Verification items for the finished model (mm, model axes). Face numbers are marked on the shaded views. A direction names the side the tool comes from. Coordinates: 2 decimals unless noted, no trailing zeros. Write each loop counter-clockwise with the first axis right and the second up, starting at its lowest first coordinate (ties: lowest second). Pieces come first, ordered by that corner, then holes. Notation, with made-up numbers: (-0.75, -10) -> (29.25, -10) arc R24 cw to (29.25, 8) -> close; hole circle Ø7 at (-0.5, -27.5). An arc over 180 degrees is marked (long way). Answer in a Markdown table with one row per item.
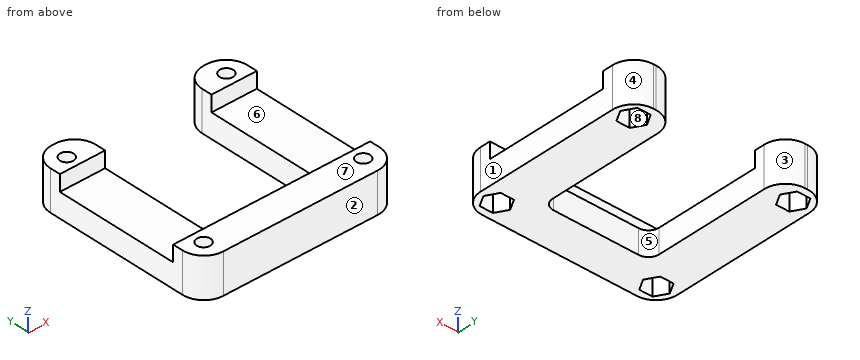
```python
from build123d import *

# Parameters (mm, degrees)
F0_R     = 1.6256
F1_DEPTH = 9.525
F2_W     = 46.99
F2_H     = 29.464
F3_DEPTH = 3.81
F5_DEPTH = 4.064


with BuildPart() as f1:
    # F0 (on Top) → F1 (new body)
    with BuildSketch(Plane.XY):
        with BuildLine():
            ThreePointArc((23.495, 17.145), (22.007102, 20.737102), (18.415, 22.225))
            Line((18.415, 22.225), (17.78, 22.225))
            ThreePointArc((17.78, 22.225), (14.187898, 20.737102), (12.7, 17.145))
            Line((12.7, 17.145), (12.7, -10.16))
            ThreePointArc((12.7, -10.16), (11.956051, -11.956051), (10.16, -12.7))
            Line((10.16, -12.7), (-10.16, -12.7))
            ThreePointArc((-10.16, -12.7), (-11.956051, -11.956051), (-12.7, -10.16))
            Line((-12.7, -10.16), (-12.7, 17.145))
            ThreePointArc((-12.7, 17.145), (-14.187898, 20.737102), (-17.78, 22.225))
            Line((-17.78, 22.225), (-18.415, 22.225))
            ThreePointArc((-18.415, 22.225), (-22.007102, 20.737102), (-23.495, 17.145))
            Line((-23.495, 17.145), (-23.495, -17.145))
            ThreePointArc((-23.495, -17.145), (-22.007102, -20.737102), (-18.415, -22.225))
            Line((-18.415, -22.225), (18.415, -22.225))
            ThreePointArc((18.415, -22.225), (22.007102, -20.737102), (23.495, -17.145))
            Line((23.495, -17.145), (23.495, 17.145))
        make_face()
        with Locations((-19.05, -17.78)):
            Circle(F0_R, mode=Mode.SUBTRACT)
        with Locations((19.05, -17.78)):
            Circle(F0_R, mode=Mode.SUBTRACT)
        with Locations((-19.05, 17.78)):
            Circle(F0_R, mode=Mode.SUBTRACT)
        with Locations((19.05, 17.78)):
            Circle(F0_R, mode=Mode.SUBTRACT)
    extrude(amount=F1_DEPTH)

    # F2 (on face) → F3 (cut)
    with BuildSketch(Plane.XY.offset(9.525)):
        Rectangle(F2_W, F2_H)
    extrude(amount=-F3_DEPTH, mode=Mode.SUBTRACT)

    # F4 (on face) → F5 (cut)
    with BuildSketch(Plane(origin=(0, 0, 0), x_dir=(1, 0, 0), z_dir=(0, 0, -1))):
        Polygon((17.466213, -15.0368), (15.882425, -17.78), (17.466213, -20.5232), (20.633787, -20.5232), (22.217575, -17.78), (20.633787, -15.0368), align=None)
        Polygon((-17.466213, -15.0368), (-20.633787, -15.0368), (-22.217575, -17.78), (-20.633787, -20.5232), (-17.466213, -20.5232), (-15.882425, -17.78), align=None)
        Polygon((15.882425, 17.78), (17.466213, 15.0368), (20.633787, 15.0368), (22.217575, 17.78), (20.633787, 20.5232), (17.466213, 20.5232), align=None)
        Polygon((-22.217575, 17.78), (-20.633787, 15.0368), (-17.466213, 15.0368), (-15.882425, 17.78), (-17.466213, 20.5232), (-20.633787, 20.5232), align=None)
    extrude(amount=-F5_DEPTH, mode=Mode.SUBTRACT)


solid = f1.part
```
1. Material ranges on probe 1 along Y at (x, z) = (-19.05, 7.3); probe 2 along X at (y, z) = (17.78, 7.25); probe 3 along X at (y, z) = (4.5, 2) (3 decimals), recorded low to high. Write a range as from..to.
Findings below:
| item | result |
|---|---|
| probe 1 | y = -22.19..-19.41, -16.15..-14.73, 14.73..16.15, 19.41..22.19 |
| probe 2 | x = -23.46..-20.68, -17.42..-12.74, 12.74..17.42, 20.68..23.46 |
| probe 3 | x = -23.495..-12.7, 12.7..23.495 |
2. Sectioned sample at D-D, the plane x = 3.5. Record the cut outline in (y, z) (3 decimals).
Findings below:
| item | result |
|---|---|
| outline | (-22.225, 0) -> (-12.7, 0) -> (-12.7, 5.715) -> (-14.732, 5.715) -> (-14.732, 9.525) -> (-22.225, 9.525) -> close |
3. Go/stop test with flat-tipped pins: pin 1 (1 mm diameter, centred on x = 19.5, z = 2.5, fed in from +Y); pin 2 (1 mm diameter, centred on x = -19.5, z = 2, fed in from -Y); pin 3 (2.5 mm diameter, centred on x = 19, y = -16.5, fed in from -Z); pin 4 (2 mm diameter, centred on x = 11.5, y = -2.5, fed in from +Z). Record where each tip stops, or that it passes through.
Findings below:
| item | result |
|---|---|
| pin 1 | stops at y = 22.19 |
| pin 2 | stops at y = -22.19 |
| pin 3 | stops at z = 4.06 |
| pin 4 | passes through |
4. Sectioned sample at B-B, the plane x = 19.05. Record the cut outline in (y, z) (3 decimals), and give its area (3 significant figures).
Findings below:
| item | result |
|---|---|
| outline | (-22.185, 0) -> (-20.523, 0) -> (-20.523, 4.064) -> (-19.406, 4.064) -> (-19.406, 9.525) -> (-22.185, 9.525) -> close; (-16.154, 4.064) -> (-15.037, 4.064) -> (-15.037, 0) -> (15.037, 0) -> (15.037, 4.064) -> (16.154, 4.064) -> (16.154, 9.525) -> (14.732, 9.525) -> (14.732, 5.715) -> (-14.732, 5.715) -> (-14.732, 9.525) -> (-16.154, 9.525) -> close; (19.406, 4.064) -> (20.523, 4.064) -> (20.523, 0) -> (22.185, 0) -> (22.185, 9.525) -> (19.406, 9.525) -> close |
| area | 230 mm² |
5. Sectioned sample at A-A, the plane y = -3.5. Record the cut outline in (x, z) (3 decimals), and give its area (3 significant figures).
Findings below:
| item | result |
|---|---|
| outline | (-23.495, 0) -> (-12.7, 0) -> (-12.7, 5.715) -> (-23.495, 5.715) -> close; (12.7, 0) -> (23.495, 0) -> (23.495, 5.715) -> (12.7, 5.715) -> close |
| area | 123 mm² |
6. Release check for a two-part mould opening along X. For the marked faces 1, 2 and 3 record: released by +X, released by -X, zero draft, split by the parting line, or undercut.
Findings below:
| item | result |
|---|---|
| face 1 | released by +X |
| face 2 | zero draft |
| face 3 | undercut |
7. Access from +Z, -Z, +X, -X, +Y, -Y to the whole of each face (thin tool, end or side, straight path). Record for the marked faces 4, 5, 6, 7 and 8.
Findings below:
| item | result |
|---|---|
| face 4 | +Z, -Z, +X, +Y |
| face 5 | +Z, -Z, +Y |
| face 6 | +Z, +X, -X |
| face 7 | +Z, +X, -X, +Y, -Y |
| face 8 | -Z |
8. Sectioned sample at C-C, the plane z = 2.5. Count the separate pieces of the cut face and the enclosed holes in it, and give its area (3 significant figures).
Findings below:
| item | result |
|---|---|
| separate pieces | 1 |
| enclosed holes | 4 |
| area | 1,070 mm² |
